```python
from build123d import *

# Parameters (mm, degrees)
F1_DEPTH = 195


with BuildPart() as f1:
    # F0 (on Front) → F1 (new body, symmetric)
    with BuildSketch(Plane.XZ):
        Polygon((319.9999762337, 305), (319.9999762337, 320), (304.9999762337, 320), (159.9999870028, 175), (174.9999875598, 160.000000557), align=None)
        Polygon((174.9999875598, 160.000000557), (159.9999870028, 175), (14.9999762337, 320), (-2.37663e-05, 320), (0, 305), (145.0000048275, 160.0000167107), (-1.114e-06, 15), (0, 0), (15, 1.114e-06), (160.0000059416, 145.0000178247), (305.0000226523, 2.26523e-05), (320, 2.37663e-05), (319.9999762337, 15.0000226523), align=None)
    extrude(amount=F1_DEPTH, both=True)


solid = f1.part
```
Design review of the part built by this model. Coordinates are the model's own, in mm. A direction names the side the tool comes from. Coordinates: 2 decimals unless noted, no trailing zeros. Loops run counter-clockwise (first coordinate to the right, second up) from the corner with the lowest first, then second, coordinate; pieces in that order, holes last. Notation, with made-up numbers: (12.5, 74) -> (50.5, 74) arc R31 ccw to (50.5, 111) -> close; hole circle Ø5 at (54, 52.25). An arc over 180 degrees is marked (long way). Answer as a JSON object with one key per item and string values.
Q1. Tool access review of faces 1 (the flat face through (249, -3, 86)), 2 (the flat face through (234, -3, 249)), 3 (the flat face through (231, -3, 74)): name each direction out of +Z, -Z, +X, -X, +Y, -Y from which nothing blocks a thin tool from reaching the whole face with its end or side.
Answer block:
{"face 1": "+X, +Y, -Y", "face 2": "+Z, +Y, -Y", "face 3": "-Z, +Y, -Y"}
Q2. To check wall thickness, follow L1, parallel to Z at x = 81.5, y = -175; L2, parallel to Z at x = 226.5, y = -131; L3, parallel to X at y = 46, z = 281. State the ranges of each line that lie inside material, in increasing order.
Answer block:
{"L1": "z = 66.5 to 96.5, 223.5 to 253.5", "L2": "z = 78.5 to 108.5, 211.5 to 241.5", "L3": "x = 24 to 54, 266 to 296"}
Q3. Clearance check with flat-ended pins moving along their axes: pin 1 Ø2 at (x, y) = (124, 110.5) entering from +Z; pin 2 Ø1 at (y, z) = (-4, 158.5) entering from -X; pin 3 Ø8 at (y, z) = (101, 272) entering from +X; pin 4 Ø4 at (x, z) = (162, 139) entering from +Y. State where each tip first meets the part, or that it passes through.
Answer block:
{"pin 1": "stops at z = 212", "pin 2": "stops at x = 143", "pin 3": "stops at x = 291", "pin 4": "passes through"}
Q4. Take a section at A-A on z = 274.5. Give the boundary of the cut face in (x, y), plus the area to 3 significant figures.
Answer block:
{"outline": "(30.5, -195) -> (60.5, -195) -> (60.5, 195) -> (30.5, 195) -> close; (259.5, -195) -> (289.5, -195) -> (289.5, 195) -> (259.5, 195) -> close", "area": "23,400 mm^2"}
Q5. The part is to be moulded in two halves that separate along Z. For faces 4 (the flat face through (246, -3, 231)), 5 (the flat face through (0, -3, 8)), 6 (the flat face through (7, -3, 0)), 7 (the flat face through (74, -3, 89)), say which applies: +Z half, -Z half, draft (parallel to the pull), parting line (faces both ways), or undercut.
Answer block:
{"face 4": "undercut", "face 5": "draft", "face 6": "-Z half", "face 7": "undercut"}
Q6. Take a section at B-B on x = 220. Give the boundary of the cut face in (y, z), plus the area to 3 significant figures.
Answer block:
{"outline": "(-195, 85) -> (195, 85) -> (195, 115) -> (-195, 115) -> close; (-195, 205) -> (195, 205) -> (195, 235) -> (-195, 235) -> close", "area": "23,400 mm^2"}
Q7. Take a section at C-C on y = -113. Give the boundary of the cut face in (x, z).
Answer block:
{"outline": "(0, 0) -> (15, 0) -> (160, 145) -> (305, 0) -> (320, 0) -> (320, 15) -> (175, 160) -> (320, 305) -> (320, 320) -> (305, 320) -> (160, 175) -> (15, 320) -> (0, 320) -> (0, 305) -> (145, 160) -> (0, 15) -> close"}
